For this review, take the finished solid that the model builds, in its own axes (mm). A direction names the side the tool comes from. Coordinates: 2 decimals unless noted, no trailing zeros. Loops run counter-clockwise (first coordinate to the right, second up) from the corner with the lowest first, then second, coordinate; pieces in that order, holes last. Notation, with made-up numbers: (51.5, 70) -> (75.5, 70) arc R28 ccw to (75.5, 108) -> close; hole circle Ø9 at (2.25, -29.75). An arc over 180 degrees is marked (long way). Use a Markdown table: item, result.
from build123d import *

# Parameters (mm, degrees)
SKETCH1_W                  = 55
SKETCH1_H                  = 65
BOSS_EXTRUDE1_DEPTH        = 10
SKETCH2_W                  = 55
SKETCH2_H                  = 5
BOSS_EXTRUDE2_DEPTH        = 15
CUT_EXTRUDE1_DEPTH         = 104
SKETCH4_W                  = 55
SKETCH4_H                  = 65
BOSS_EXTRUDE3_DEPTH        = 5
M5_TAPPED_HOLE2_AT_2_COUNT = 2
M5_TAPPED_HOLE2_AT_2_PITCH = 15
M5_TAPPED_HOLE2_AT_3_COUNT = 2
M5_TAPPED_HOLE2_AT_3_PITCH = 30
M5_TAPPED_HOLE2_AT_4_COUNT = 2
M5_TAPPED_HOLE2_AT_4_PITCH = 45
BOSS_EXTRUDE4_START        = 5
SKETCH13_W                 = 55
SKETCH13_H                 = 30
BOSS_EXTRUDE4_DEPTH        = 5
CHAMFER2_SIZE              = 1.5


with BuildPart() as part:
    # Sketch1 → Boss-Extrude1 (new body)
    with BuildSketch(Plane.XY):
        Rectangle(SKETCH1_W, SKETCH1_H)
    extrude(amount=BOSS_EXTRUDE1_DEPTH)

    # Sketch2 → Boss-Extrude2 (add)
    with BuildSketch(Plane(origin=(0, 0, 0), x_dir=(-1, 0, 0), z_dir=(0, 0, -1))):
        with Locations((0, 30)):
            Rectangle(SKETCH2_W, SKETCH2_H)
        with Locations((0, -30)):
            Rectangle(SKETCH2_W, SKETCH2_H)
    extrude(amount=BOSS_EXTRUDE2_DEPTH)

    # Sketch3 → Cut-Extrude1 (cut)
    with BuildSketch(Plane.XZ.offset(32.5)):
        with BuildLine():
            Line((-20.05, -4.75), (19.95, -4.75))
            ThreePointArc((19.95, -4.75), (22.7, -7.5), (19.95, -10.25))
            Line((19.95, -10.25), (-20.05, -10.25))
            ThreePointArc((-20.05, -10.25), (-22.8, -7.5), (-20.05, -4.75))
        make_face()
    extrude(amount=-CUT_EXTRUDE1_DEPTH, mode=Mode.SUBTRACT)

    # Sketch4 → Boss-Extrude3 (add)
    with BuildSketch(Plane.XY.offset(10)):
        Rectangle(SKETCH4_W, SKETCH4_H)
    extrude(amount=BOSS_EXTRUDE3_DEPTH)

    # Sketch12 → M5 Tapped Hole2 (revolve, cut)
    with BuildSketch(Plane(origin=(27.5, 22.5, 7.5), x_dir=(0, 0, -1), z_dir=(0, 1, 0))):
        Polygon((0, 0), (0, 15.2618073), (2.1, 14), (2.1, 0), align=None)
    m5_tapped_hole2 = revolve(axis=Axis((33.85, 22.5, 7.5), (-1, 0, 0)), mode=Mode.SUBTRACT)

    # M5 Tapped Hole2 at 2: M5 Tapped Hole2 ×2
    with Locations(*[(0, -i * M5_TAPPED_HOLE2_AT_2_PITCH, 0) for i in range(1, M5_TAPPED_HOLE2_AT_2_COUNT)]):
        add(m5_tapped_hole2, mode=Mode.SUBTRACT)

    # M5 Tapped Hole2 at 3: M5 Tapped Hole2 ×2
    with Locations(*[(0, -i * M5_TAPPED_HOLE2_AT_3_PITCH, 0) for i in range(1, M5_TAPPED_HOLE2_AT_3_COUNT)]):
        add(m5_tapped_hole2, mode=Mode.SUBTRACT)

    # M5 Tapped Hole2 at 4: M5 Tapped Hole2 ×2
    with Locations(*[(0, -i * M5_TAPPED_HOLE2_AT_4_PITCH, 0) for i in range(1, M5_TAPPED_HOLE2_AT_4_COUNT)]):
        add(m5_tapped_hole2, mode=Mode.SUBTRACT)

    # Mirror2: M5 Tapped Hole2 across plane
    add(m5_tapped_hole2.mirror(Plane(origin=(0, 0, 0), x_dir=(0, 0, 1), z_dir=(1, 0, 0))), mode=Mode.SUBTRACT)

    # Mirror2 copy 1 sketch → Mirror2 copy 1 (revolve, cut)
    with BuildSketch(Plane(origin=(-27.5, 7.5, 7.499975629), x_dir=(0, 0, -1), z_dir=(0, 1, 0))):
        Polygon((0, 0), (0, -15.2618073), (2.1, -14), (2.1, 0), align=None)
    revolve(axis=Axis((-33.85, 7.5, 7.499975629), (-1, 0, 0)), mode=Mode.SUBTRACT)

    # Mirror2 copy 2 sketch → Mirror2 copy 2 (revolve, cut)
    with BuildSketch(Plane(origin=(-27.5, -7.5, 7.499949533), x_dir=(0, 0, -1), z_dir=(0, 1, 0))):
        Polygon((0, 0), (0, -15.2618073), (2.1, -14), (2.1, 0), align=None)
    revolve(axis=Axis((-33.85, -7.5, 7.499949533), (-1, 0, 0)), mode=Mode.SUBTRACT)

    # Mirror2 copy 3 sketch → Mirror2 copy 3 (revolve, cut)
    with BuildSketch(Plane(origin=(-27.5, -22.5, 7.499923436), x_dir=(0, 0, -1), z_dir=(0, 1, 0))):
        Polygon((0, 0), (0, -15.2618073), (2.1, -14), (2.1, 0), align=None)
    revolve(axis=Axis((-33.85, -22.5, 7.499923436), (-1, 0, 0)), mode=Mode.SUBTRACT)

    # Sketch13 → Boss-Extrude4 (add)
    with BuildSketch(Plane.XZ.offset(32.5).offset(BOSS_EXTRUDE4_START)):
        Rectangle(SKETCH13_W, SKETCH13_H)
        with BuildLine():
            Line((-20.05, -4.75), (19.95, -4.75))
            ThreePointArc((19.95, -4.75), (22.7, -7.5), (19.95, -10.25))
            Line((19.95, -10.25), (-20.05, -10.25))
            ThreePointArc((-20.05, -10.25), (-22.8, -7.5), (-20.05, -4.75))
        make_face(mode=Mode.SUBTRACT)
    boss_extrude4 = extrude(amount=-BOSS_EXTRUDE4_DEPTH)

    # Mirror3: Boss-Extrude4 across plane
    add(boss_extrude4.mirror(Plane(origin=(0, 0, 0), x_dir=(0, 0, 1), z_dir=(0, -1, 0))))

    # Chamfer2
    chamfer2_edges = [part.edges().sort_by_distance(p)[0] for p in [
        (-27.5, -37.5, 0),
        (0, -37.5, -15),
        (27.5, -37.5, 0),
        (0, -37.5, 15),
        (-27.5, 37.5, 0),
        (0, 37.5, 15),
        (27.5, 37.5, 0),
        (0, 37.5, -15),
        (27.5, 32.5, -15),
        (-27.5, 32.5, -15),
        (27.5, -32.5, -15),
        (-27.5, -32.5, -15),
        (-27.5, 0, 15),
        (27.5, 0, 15),
    ]]
    chamfer(chamfer2_edges, length=CHAMFER2_SIZE)


solid = part.part
(1) Take a section at C-C on z = -1.25. Write out the cut boundary in (x, y).
Found:
| item | result |
|---|---|
| outline | (-27.5, -36) -> (-26, -37.5) -> (26, -37.5) -> (27.5, -36) -> (27.5, -27.5) -> (-27.5, -27.5) -> close; (-27.5, 27.5) -> (27.5, 27.5) -> (27.5, 36) -> (26, 37.5) -> (-26, 37.5) -> (-27.5, 36) -> close |
(2) For pin 1 Ø2.5 at (y, z) = (-7.5, 7.5) entering from -X; pin 2 Ø6 at (x, y) = (-11.5, 21) entering from -Z; pin 3 Ø2.5 at (y, z) = (-22.5, 7.5) entering from +X, all flat-tipped, find the tip position at first contact; note any pin that passes through.
Found:
| item | result |
|---|---|
| pin 1 | stops at x = -12.99 |
| pin 2 | stops at z = 0 |
| pin 3 | stops at x = 12.99 |
(3) For line 1 along Y through (x, z) = (20.75, 7.5); line 2 along Y through (x, z) = (-9, -3.5); line 3 along Z through (x, y) = (18, -32.5), list the stretches that pass through material, from the lowest coordinate up.
Found:
| item | result |
|---|---|
| line 1 | y = -37.5 to -24.6, -20.4 to -9.6, -5.4 to 5.4, 9.6 to 20.4, 24.6 to 37.5 |
| line 2 | y = -37.5 to -27.5, 27.5 to 37.5 |
| line 3 | z = -15 to -10.25, -4.75 to 15 |
(4) Take a section at D-D on x = 3.5. Write out the cut boundary in (y, z), plus the area to 3 significant figures.
Found:
| item | result |
|---|---|
| outline | (-37.5, -13.5) -> (-36, -15) -> (-27.5, -15) -> (-27.5, -10.25) -> (-37.5, -10.25) -> close; (-37.5, -4.75) -> (-27.5, -4.75) -> (-27.5, 0) -> (27.5, 0) -> (27.5, -4.75) -> (37.5, -4.75) -> (37.5, 13.5) -> (36, 15) -> (-36, 15) -> (-37.5, 13.5) -> close; (27.5, -15) -> (36, -15) -> (37.5, -13.5) -> (37.5, -10.25) -> (27.5, -10.25) -> close |
| area | 1,310 mm^2 |
(5) Take a section at A-A on z = -7.5. Write out the cut boundary in (x, y), plus the area to 4 significant figures.
Found:
| item | result |
|---|---|
| outline | (-27.5, -36) -> (-26, -37.5) -> (-22.8, -37.5) -> (-22.8, -27.5) -> (-27.5, -27.5) -> close; (-27.5, 27.5) -> (-22.8, 27.5) -> (-22.8, 37.5) -> (-26, 37.5) -> (-27.5, 36) -> close; (22.7, -37.5) -> (26, -37.5) -> (27.5, -36) -> (27.5, -27.5) -> (22.7, -27.5) -> close; (22.7, 27.5) -> (27.5, 27.5) -> (27.5, 36) -> (26, 37.5) -> (22.7, 37.5) -> close |
| area | 185.5 mm^2 |
(6) Mouldability with a two-part tool opening along X and no side actions: class faces 6 (the face through (12.46, 22.86, 7.58)), 7 (the face through (0, 27.5, -4)), 8 (the face through (22.7, 32.6, -7.4)) as pulls with the +X half, pulls with the -X half, needs draft (parallel to the pull), parting line crosses it, or undercut.
Found:
| item | result |
|---|---|
| face 6 | pulls with the +X half |
| face 7 | needs draft |
| face 8 | undercut |
(7) For faces 1 (the face through (-12.46, -7.75, 7.77)), 2 (the face through (0, -33, -4.75)), 3 (the face through (20.598, 5.418, 7.773)), 4 (the face through (0, 0, 0)), 5 (the face through (-26.453, 36.474, -14.073)), list the 3-axis set-ups (+Z, -Z, +X, -X, +Y, -Y) from which the entire face can be reached by the end or side of a thin tool; tool diameter is ignored.
Found:
| item | result |
|---|---|
| face 1 | -X |
| face 2 | +Y, -Y |
| face 3 | +X |
| face 4 | -Z, +X, -X |
| face 5 | -Z, -X, +Y |
(8) Take a section at B-B on x = 14.5. Write out the cut boundary in (y, z), plus the area to 3 significant figures.
Found:
| item | result |
|---|---|
| outline | (-37.5, -13.5) -> (-36, -15) -> (-27.5, -15) -> (-27.5, -10.25) -> (-37.5, -10.25) -> close; (-37.5, -4.75) -> (-27.5, -4.75) -> (-27.5, 0) -> (27.5, 0) -> (27.5, -4.75) -> (37.5, -4.75) -> (37.5, 13.5) -> (36, 15) -> (-36, 15) -> (-37.5, 13.5) -> close; (27.5, -15) -> (36, -15) -> (37.5, -13.5) -> (37.5, -10.25) -> (27.5, -10.25) -> close; hole circle Ø4.2 at (-22.5, 7.5); hole circle Ø4.2 at (-7.5, 7.5); hole circle Ø4.2 at (7.5, 7.5); hole circle Ø4.2 at (22.5, 7.5) |
| area | 1,260 mm^2 |
